Autodesk Inventor part; units mm, degrees
ref_plane "YZ Plane" through (0, 0, 0) normal (1, 0, 0) x (0, 1, 0)
ref_plane "XZ Plane" through (0, 0, 0) normal (0, 1, 0) x (-1, 0, 0)
ref_plane "XY Plane" through (0, 0, 0) normal (0, 0, 1) x (1, 0, 0)
sketch "スケッチ1" plane through (0, 0, 0) normal (0, 1, 0) x (-1, 0, 0)
  arc A0 (348.9954, -50.1786) -> (348.3553, -42.2361) centre (348.3204, -46.2359) ccw
  arc A1 (182.359, -65.8653) -> (348.9954, -50.1786) centre (162.2533, 1040.6287) ccw
  arc A2 (135.1603, -65.3257) -> (182.359, -65.8653) centre (167.871, 731.467) ccw
  arc A3 (48.4731, -49.9165) -> (135.1603, -65.3257) centre (148.588, 261.756) ccw
  arc A4 (-1.5687, -25.3375) -> (48.4731, -49.9165) centre (107.173, 132.825) ccw
  arc A5 (-15.7749, -11.5429) -> (-1.5687, -25.3375) centre (31.9, 23.342) ccw
  arc A6 (-8.2474, 11.5993) -> (-15.7749, -11.5429) centre (-3.6695, -2.6851) ccw
  arc A7 (13.0537, 14.3873) -> (-8.2474, 11.5993) centre (10.0641, -45.5382) ccw
  arc A8 (91.047, 0) -> (13.0537, 14.3873) centre (-1.8944, -285.2401) ccw
  arc A9 (91.047, 0) -> (95.8009, -1.5381) centre (462.8125, 1140.9603) ccw
  arc A10 (95.8009, -1.5381) -> (348.3553, -42.2361) centre (355.7675, 807.7316) ccw
  point P0 (0, 0)
extrude "押し出し1" add sketch "スケッチ1" along normal mid plane 4
sketch "スケッチ2" plane through (0, -2, 0) normal (0, -1, 0) x (1, 0, 0)
  line L0 (0, 0) -> (-283.8627, -59.346)
  arc A0 (-348.9954, -50.1786) -> (-182.359, -65.8653) centre (-162.2533, 1040.6287) ccw
  circle A1 centre (-29.3651, -6.1392) radius 6
  circle A2 centre (-239.8151, -50.1371) radius 6
  dimension "d3" = 290
  dimension "d4" = 12
  dimension "d5" = 12
  dimension "d6" = 30
  dimension "d7" = 215
extrude "押し出し2" cut sketch "スケッチ2" against normal through all
thicken "厚み1" operation cut thickness 3 both sides no extend neighbours no toward (0.1519877, 0, -0.9883824) faces at (-226.5779, 0.6667, -32.3934) (-92.1028, 0.6667, -0.3435) (-19.6698, -0.6667, 13.9839) (-3.4686, 0.6667, 14.0982) (9.3583, 0.6667, 11.1943) (14.4364, 0.6667, -13.3021) (-19.7763, 0.6667, -38.0608) (-76.8673, 0.6667, -57.648) (-177.1142, -0.6667, -65.9433) (-238.1449, 0.6667, -63.4427) (-351.8388, 0.6667, -48.1388)
properties part number "flap_m" material "木材 (オーク)"
Check sheet for the modelled part. Datum: model origin and axes. Units: mm. Coordinates: 2 decimals unless noted, no trailing zeros. Loops run counter-clockwise (first coordinate to the right, second up) from the corner with the lowest first, then second, coordinate; pieces in that order, holes last. Notation, with made-up numbers: (-33.75, 79) -> (8.25, 79) arc R22 ccw to (8.25, 117) -> close; hole circle Ø4 at (29, -14). An arc over 180 degrees is marked (long way). Write item = value, one per line. Start each with the question number.
1. Depth check by flat-ended pin: P1, Ø2, axis at x = -271.5, z = -40, coming from the +Y side. Enter the tip coordinate at first touch or a pass-through.
2. Section check A-A on y = -0.95. Record the cut outline in (x, z).
3. Material ranges on line 1 (Z direction, x = -331.5, y = 1.2); line 2 (Z direction, x = -149, y = -1.8), recorded low to high.
4. Section check B-B on z = -36. Record the cut outline in (x, y).
5. Draft check along Z on faces 1 (the flat face through (-124, -2, -34)), 2 (the cylindrical face through (-24.22, -0.03, -36.93)), 3 (the cylindrical face through (-51.44, -0.03, 6.93)), 4 (the cylindrical face through (-34.126, -0.028, -9.79)). Enter one of: released by +Z, released by -Z, zero draft, split by the parting line, or undercut.
6. Section check C-C on x = -192. Record the cut outline in (y, z), then the cut area to 3 significant figures.
Responses:
q1.P1 = through
q2.outline = (-348.49, -47.22) arc R1103.67 ccw to (-182.3, -62.87) arc R794.54 ccw to (-135.28, -62.33) arc R324.36 ccw to (-49.39, -47.06) arc R188.94 ccw to (-0.13, -22.87) arc R56.07 ccw to (13.35, -9.77) arc R12 ccw to (7.33, 8.74) arc R57 ccw to (-12.9, 11.39) arc R297 ccw to (-90.12, -2.85) arc R1214.19 cw to (-94.88, -4.39) arc R853 cw to (-348.33, -45.24) arc R1 ccw to start; hole circle Ø12 at (-239.82, -50.14); hole circle Ø12 at (-29.37, -6.14)
q3.line_1 = -49.99 to -44.92
q3.line_2 = -62.77 to -19.83
q4.outline = (-230.36, -2) -> (-22.35, -2) -> (-22.35, 2) -> (-230.36, 2) -> close
q5.face_1 = zero draft
q5.face_2 = released by -Z
q5.face_3 = released by +Z
q5.face_4 = undercut
q6.outline = (-2, -62.65) -> (2, -62.65) -> (2, -29.4) -> (-2, -29.4) -> close
q6.area = 133 mm2
